Could you check a few things on this model? Use its own coordinates, in mm. Face numbers are marked on the shaded views. A direction names the side the tool comes from. Give positions to 0.01 mm unless a question says otherwise; leave off trailing zeros. Write each loop counter-clockwise with the first axis right and the second up, starting at its lowest first coordinate (ties: lowest second). Pieces come first, ordered by that corner, then holes. Notation, with made-up numbers: M 66.25,33 L 108.25,33 A13 cw 108.25,51 Z; hole C 28,22.25 d4. An arc over 180 degrees is marked long. Answer as a JSON object with one key per item and string values. Group by question number.
Solid Edge part; units mm, degrees
sketch "Sketch1" plane through (0, 0, 0) normal (0, -1, 0) x (1, 0, 0)
  line L0 (-5.3694, 18.9) -> (-19.0694, -4.8291)
  arc A0 (-13.7, -14.1291) -> (-19.0694, -4.8291) centre (-13.7, -7.9291) cw
  line L1 (-13.7, -14.1291) -> (13.7, -14.1291)
  arc A1 (19.0694, -4.8291) -> (13.7, -14.1291) centre (13.7, -7.9291) cw
  line L2 (5.3694, 18.9) -> (19.0694, -4.8291)
  arc A2 (-5.3694, 18.9) -> (5.3694, 18.9) centre (0, 15.8) cw
  dimension "D1" = 5.3694
extrude "Protrusion1" add sketch "Sketch1" against normal blind 14
sketch "Sketch2" plane through (0, 0, 0) normal (0, -1, 0) x (1, 0, 0)
  circle A0 centre (-13.7, -7.9291) radius 2.2
  circle A1 centre (13.7, -7.9291) radius 2.2
  circle A2 centre (0, 15.8) radius 2.2
extrude "Cutout1" cut sketch "Sketch2" against normal blind 457.8755
sketch "Sketch3" plane through (0, 0, 0) normal (0, -1, 0) x (1, 0, 0)
  circle A0 centre (0, 0) radius 9.3
extrude "Cutout2" cut sketch "Sketch3" against normal blind 434.4917
sketch "Sketch4" plane through (0, 0, 3.9355) normal (0, -1, 0) x (-0.5, 0, 0.8660254)
  line L0 (-23.325, -5.9323) -> (-23.325, -18.9323)
  line L1 (-23.325, -18.9323) -> (16.475, -18.9323)
  line L2 (16.475, -18.9323) -> (16.475, -5.9323)
  line L3 (12.7755, -8.7037) -> (16.475, -5.9323)
  line L4 (-20.9306, -8.7037) -> (12.7755, -8.7037)
  line L5 (-20.9306, -5.9323) -> (-20.9306, -8.7037)
  line L6 (-23.325, -5.9323) -> (-20.9306, -5.9323)
  dimension "D1" = 23.325
extrude "Protrusion2" add sketch "Sketch4" against normal up to vertex (14 mm away)
sketch "Sketch5" plane through (18.1083, 8, 10.4355) normal (0.8660254, 0, 0.5) x (-0.5, 0, 0.8660254)
  line L0 (-19.9, 8) -> (19.9, 8)
  line L1 (19.9, -6) -> (19.9, 8)
  line L2 (-19.9, -6) -> (19.9, -6)
  line L3 (-19.9, -6) -> (-19.9, 8)
extrude "ExtrudedProtrusion_14" add sketch "Sketch5" along normal blind 4
sketch "Sketch6" plane through (5.8112, 14, 7.7701) normal (0, 1, 0) x (0.5, 0, -0.8660254)
  circle A0 centre (3.8403, 24.7468) radius 3.7
  circle A1 centre (17.5403, 1.0177) radius 3.7
  circle A2 centre (-9.8597, 1.0177) radius 3.7
extrude "Cutout3" cut sketch "Sketch6" against normal blind 8
sketch "Sketch7" plane through (11.8615, 14, 7.7701) normal (0, 1, 0) x (-0.8660254, 0, -0.5)
  circle A0 centre (-2.5426, -0.8152) radius 2.2
extrude "ExtrudedCutout_23" cut sketch "Sketch7" against normal blind 166.5817
sketch "Sketch8" plane through (11.8615, 14, 7.7701) normal (0, 1, 0) x (-0.8660254, 0, -0.5)
  circle A0 centre (40.6865, -0.8152) radius 2.2
  line L0 (40.6865, 5.6848) -> (31.1282, 5.6848)
  line L1 (31.1282, 5.6848) -> (31.1282, 3.8832)
  line L2 (31.1282, 3.8832) -> (34.2429, 1.8592)
  line L3 (34.2429, 1.8592) -> (34.2429, -2.6486)
  line L4 (31.1282, -7.3152) -> (34.2429, -2.6486)
  line L5 (40.6865, -7.3152) -> (31.1282, -7.3152)
  arc A1 (40.6865, -7.3152) -> (40.6865, 5.6848) centre (40.6865, -0.8152) ccw
extrude "Protrusion3" add sketch "Sketch8" against normal up to vertex (14 mm away)
sketch "Sketch9" plane through (11.8615, 14, 7.7701) normal (0, 1, 0) x (-0.8660254, 0, -0.5)
  line L0 (-10.7426, -0.8152) -> (-10.7426, -20.7152)
  line L1 (-10.7426, -20.7152) -> (6.2574, -20.7152)
  arc A0 (1.1563, -18.0392) -> (6.2574, -20.7152) centre (6.2574, -14.5152) ccw
  line L2 (1.1563, -18.0392) -> (-10.7426, -0.8152)
extrude "Cutout4" cut sketch "Sketch9" against normal blind 85.4791
sketch "Sketch10" plane through (6.8865, 14, 7.7701) normal (0, 1, 0) x (-0.8660254, 0, -0.5)
  line L0 (-15.0511, 16.5973) -> (-15.0511, -3.3027)
  line L1 (-3.1522, 13.9213) -> (-15.0511, -3.3027)
  arc A0 (1.9489, 16.5973) -> (-3.1522, 13.9213) centre (1.9489, 10.3973) ccw
  line L2 (1.9489, 16.5973) -> (-15.0511, 16.5973)
extrude "ExtrudedCutout_27" cut sketch "Sketch10" against normal blind 118.3722
sketch "Sketch11" plane through (0, 0, 0) normal (0, 0, 1) x (1, 0, 0)
  line L0 (-57, 0) -> (32.4619, 0)
  line L1 (32.4619, 0) -> (32.4619, 3)
  line L2 (32.4619, 3) -> (-57, 3)
  line L3 (-57, 3) -> (-57, 0)
  dimension "D1" = 57
extrude "Cutout5" cut sketch "Sketch11" along normal mid plane 82.8276
sketch "Sketch12" plane through (11.8615, 14, 7.7701) normal (0, 1, 0) x (-0.8660254, 0, -0.5)
  line L0 (2.6574, 7.7016) -> (2.6574, -9.2984)
  line L1 (2.6574, -9.2984) -> (7.9574, -15.2984)
  arc A0 (20.3574, -15.2984) -> (7.9574, -15.2984) centre (14.1574, -9.8217) cw
  line L2 (25.6574, -9.2984) -> (20.3574, -15.2984)
  line L3 (25.6574, 7.7016) -> (25.6574, -9.2984)
  line L4 (25.6574, 7.7016) -> (20.3574, 13.7016)
  arc A1 (7.9574, 13.7016) -> (20.3574, 13.7016) centre (14.1574, 8.2249) cw
  line L5 (2.6574, 7.7016) -> (7.9574, 13.7016)
extrude "Cutout6" cut sketch "Sketch12" against normal blind 3.8
fillet "Round_2" radius 5 1 edges at (21.5724, 8.5, 12.4355)
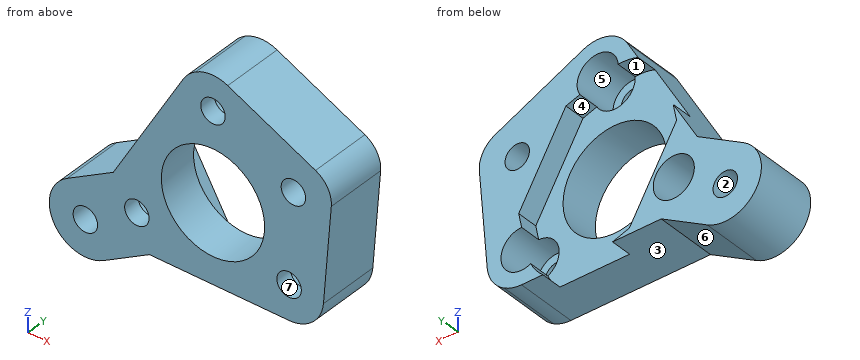
1) We'd pull the mould along X, two halves only. Please class the marked faces 4, 5, 6 and 7: released by +X, released by -X, zero draft, split by the parting line, or undercut.
2) For the marked faces 1, 2 and 3, which set-ups out of +Z, -Z, +X, -X, +Y, -Y let a thin tool reach every point of the face, with its end or its side?
3) If we section it at D-D, the plane x = 8: List the corners of the cut face in (y, z) for me.
4) If we section it at B-B, the plane z = 4: List the corners of the cut face in (x, y) for me, plus the area to 3 significant figures.
5) Please list where these lines run through material, in increasing order: line 1 along Z through (x, y) = (0, 3.75); line 2 along Z through (x, y) = (13.7, 3.85); line 3 along X through (y, z) = (7, -9.5). Write a range as from..to.
6) I'm going to push flat-ended pins straight in: pin 1 (3.5 mm diameter, centred on x = 14.5, z = -7, fed in from +Y); pin 2 (1 mm diameter, centred on x = 15.5, y = 12, fed in from +Z); pin 3 (1.5 mm diameter, centred on y = 5, z = 14, fed in from -X). Where does each tip first touch, or does it pass through?
7) If we section it at A-A, the plane x = 0: List the corners of the cut face in (y, z) for me, plus the area to 3 significant figures.
Taken from the geometry:
{
 "1": {"face 4": "released by -X", "face 5": "undercut", "face 6": "released by +X", "face 7": "undercut"},
 "2": {"face 1": "+Y", "face 2": "+Y, -Y", "face 3": "-Z, +X, +Y, -Y"},
 "3": {"outline": "M 3,-14.13 L 10.2,-14.13 L 10.2,-4.74 L 3,-4.74 Z; M 3,4.74 L 10.2,4.74 L 10.2,9.14 L 14,9.14 L 14,18.87 L 3,18.87 Z"},
 "4": {"outline": "M -13.97,3 L -8.4,3 L -8.4,10.2 L -13.73,10.2 L -13.73,14 L -13.97,14 Z; M 8.4,3 L 20.89,3 L 20.89,14 L 10.97,14 L 10.97,10.2 L 8.4,10.2 Z", "area": "169 mm²"},
 "5": {"line 1": "-14.13..-9.3, 9.3..13.6, 18..22", "line 2": "-14.13..-10.13, -5.73..6.27, 10.4..16.17", "line 3": "-28.25..-17.05, -10.35..10.35, 17.05..19.7"},
 "6": {"pin 1": "y = 6", "pin 2": "z = 15.55", "pin 3": "x = -8.63"},
 "7": {"outline": "M 3,-14.13 L 10.2,-14.13 L 10.2,-9.3 L 3,-9.3 Z; M 3,9.3 L 10.2,9.3 L 10.2,12.1 L 6,12.1 L 6,13.6 L 3,13.6 Z; M 3,18 L 6,18 L 6,19.5 L 14,19.5 L 14,22 L 3,22 Z", "area": "91.4 mm²"}
}
